from build123d import *

# Parameters (mm, degrees)
SALIENTE_EXTRUIR1_DEPTH = 0.1


with BuildPart() as part:
    # Model → Saliente-Extruir1 (new body)
    with BuildSketch(Plane.XY):
        with BuildLine():
            Line((46.781292642, 16.163412143), (45.210633071, 9.597207197))
            ThreePointArc((45.210633071, 9.597207197), (46.428733439, 10.136393874), (47.745640238, 9.935776663))
            ThreePointArc((47.745640238, 9.935776663), (48.227185328, 8.874486831), (48.29361035, 7.710953635))
            ThreePointArc((48.29361035, 7.710953635), (46.29339053, 0.212855495), (41.414561099, -5.821991516))
            Line((41.414561099, -5.821991516), (40.94311821, -7.574533899))
            Line((40.94311821, -7.574533899), (51.874825524, -9.299930098))
            Line((51.874825524, -9.299930098), (45.610263372, -4.601508484))
            Line((45.610263372, -4.601508484), (53.387805188, -7.231700789))
            Line((53.387805188, -7.231700789), (49.78663814, 2.533131744))
            ThreePointArc((49.78663814, 2.533131744), (53.21025646, 11.68516332), (62.108805747, 15.722076119))
            ThreePointArc((62.108805747, 15.722076119), (58.405273393, 19.222364472), (53.363625788, 18.480771672))
            ThreePointArc((53.363625788, 18.480771672), (59.163542766, 23.716796233), (66.656485293, 25.932829273))
            ThreePointArc((66.656485293, 25.932829273), (59.050669494, 25.500073296), (52.661184456, 21.351556375))
            ThreePointArc((52.661184456, 21.351556375), (47.085279202, 29.377399858), (38.526658627, 34.094909461))
            ThreePointArc((38.526658627, 34.094909461), (31.0230825, 51.465775367), (13.185822242, 57.781057111))
            ThreePointArc((13.185822242, 57.781057111), (17.428790822, 46.402823396), (11.027622368, 36.083325964))
            ThreePointArc((11.027622368, 36.083325964), (6.141614269, 41.955490113), (-0.549240207, 45.641660661))
            ThreePointArc((-0.549240207, 45.641660661), (-6.565835805, 44.626508675), (-11.474115224, 41.001767403))
            ThreePointArc((-11.474115224, 41.001767403), (-3.043112078, 38.133520464), (0.430717912, 29.933449747))
            ThreePointArc((0.430717912, 29.933449747), (-6.1199859, 29.496958972), (-11.558821293, 25.819825005))
            ThreePointArc((-11.558821293, 25.819825005), (-7.516746047, 21.932992962), (-5.013290934, 16.915169916))
            ThreePointArc((-5.013290934, 16.915169916), (-4.924563846, 19.307742761), (-3.862473188, 21.453492221))
            ThreePointArc((-3.862473188, 21.453492221), (-1.404763761, 24.311648506), (1.453102003, 26.769695749))
            ThreePointArc((1.453102003, 26.769695749), (4.666243247, 23.605511541), (9.078509713, 22.673715965))
            ThreePointArc((9.078509713, 22.673715965), (6.210508457, 25.484631427), (5.747363145, 29.473637989))
            ThreePointArc((5.747363145, 29.473637989), (10.121021769, 31.249866453), (14.765165078, 32.095922149))
            ThreePointArc((14.765165078, 32.095922149), (15.665979392, 23.525430747), (18.59573809, 15.421030506))
            ThreePointArc((18.59573809, 15.421030506), (21.47392467, 25.106483656), (29.012326443, 31.834370355))
            ThreePointArc((29.012326443, 31.834370355), (33.11905298, 31.270823266), (37.01078738, 29.843521077))
            ThreePointArc((37.01078738, 29.843521077), (36.737947796, 24.937066035), (34.858893184, 20.396482781))
            ThreePointArc((34.858893184, 20.396482781), (38.209567477, 23.825829531), (39.356591195, 28.481124787))
            ThreePointArc((39.356591195, 28.481124787), (40.05251455, 28.065666009), (40.657061832, 27.525816125))
            ThreePointArc((40.657061832, 27.525816125), (40.534478216, 23.70157311), (39.613613517, 19.987832464))
            ThreePointArc((39.613613517, 19.987832464), (41.978685113, 21.980935805), (43.538467404, 24.651722914))
            ThreePointArc((43.538467404, 24.651722914), (45.261167282, 22.234594253), (46.637218774, 19.604634534))
            ThreePointArc((46.637218774, 19.604634534), (46.937945055, 17.893597889), (46.781292642, 16.163412143))
        make_face()
    extrude(amount=SALIENTE_EXTRUIR1_DEPTH)


solid = part.part
Can you work these out from the model? Positions are in its coordinate system, mm. Coordinates: 2 decimals unless noted, no trailing zeros. Loops run counter-clockwise (first coordinate to the right, second up) from the corner with the lowest first, then second, coordinate; pieces in that order, holes last. Notation, with made-up numbers: (35, 44) - (91, 44) arc R16 cw to (91, 68) - close; hole circle Ø10 at (48.25, 60.25). An arc over 180 degrees is marked (long way). Put each result on its own line as item: value. Start each with the question number.
Item 1: Suppose I cut it at D-D (x = 22). Please give me the cut outline in (y, z), and give its area (3 significant figures).
Item 2: Suppose I cut it at B-B (y = 43). Please give me the cut outline in (x, z), and give its area (3 significant figures).
Item 3: If I drill on line 1 along X through (y, z) = (18, 0.05); line 2 along Y through (x, z) = (12, 0.05); line 3 along X through (y, z) = (46, 0.05), over which ranges is the centre line in solid material (lowest first)?
Item 4: Suppose I cut it at A-A (x = -2). Please give me the cut outline in (y, z).
Item 5: Suppose I cut it at C-C (y = 1). Please give me the cut outline in (x, z), and give its area (3 significant figures).
Here are the results:
1. outline: (25.89, 0) - (56.74, 0) - (56.74, 0.1) - (25.89, 0.1) - close
1. area: 3.08 mm²
2. outline: (-9.37, 0) - (4.76, 0) - (4.76, 0.1) - (-9.37, 0.1) - close; (16.65, 0) - (36.82, 0) - (36.82, 0.1) - (16.65, 0.1) - close
2. area: 3.43 mm²
3. line 1: -5.38 to -5.1, 17.42 to 18.81, 46.93 to 60.55
3. line 2: 31.71 to 36.75
3. line 3: 17.38 to 35.36
4. outline: (23.7, 0) - (30.18, 0) - (30.18, 0.1) - (23.7, 0.1) - close; (37.02, 0) - (45.66, 0) - (45.66, 0.1) - (37.02, 0.1) - close
5. outline: (46.67, 0) - (50.35, 0) - (50.35, 0.1) - (46.67, 0.1) - close
5. area: 0.368 mm²
